```python
from build123d import *

# Parameters (mm, degrees)
SKETCH2_W     = 0.9
SKETCH2_H     = 0.2
CHAMFER1_SIZE = 0.8
CHAMFER2_SIZE = 0.3


with BuildPart() as part:
    # Sketch1 → Revolve1 (revolve)
    with BuildSketch(Plane(origin=(0, 0, 0), x_dir=(0, 0, -1), z_dir=(1, 0, 0)), mode=Mode.PRIVATE) as revolve1_sk:
        Polygon((-150, 0), (150, 0), (150, 4), (140, 4), (140, 6.32), (-96, 6.32), (-96, 4.94), (-135, 4.94), (-135, 4), (-150, 4), align=None)
    revolve(revolve1_sk.sketch.rotate(Axis((0, 0, 150), (0, 0, -1)), 90), axis=Axis((0, 0, 150), (0, 0, -1)))

    # Sketch2 → Cut-Revolve1 (revolve, cut)
    with BuildSketch(Plane(origin=(0, 0, 0), x_dir=(0, 0, -1), z_dir=(1, 0, 0)), mode=Mode.PRIVATE) as cut_revolve1_sk:
        with Locations((147.45, 3.9)):
            Rectangle(SKETCH2_W, SKETCH2_H)
    revolve(cut_revolve1_sk.sketch.rotate(Axis((0, 0, -150), (0, 0, 1)), 270), axis=Axis((0, 0, -150), (0, 0, 1)), mode=Mode.SUBTRACT)

    # Chamfer1
    chamfer1_edges = [part.edges().sort_by_distance(p)[0] for p in [
        (-4, 0, -150),
    ]]
    chamfer(chamfer1_edges, length=CHAMFER1_SIZE)

    # Chamfer2
    chamfer2_edges = [part.edges().sort_by_distance(p)[0] for p in [
        (-4.94, 0, 135),
        (-4, 0, 150),
    ]]
    chamfer(chamfer2_edges, length=CHAMFER2_SIZE)


solid = part.part
```
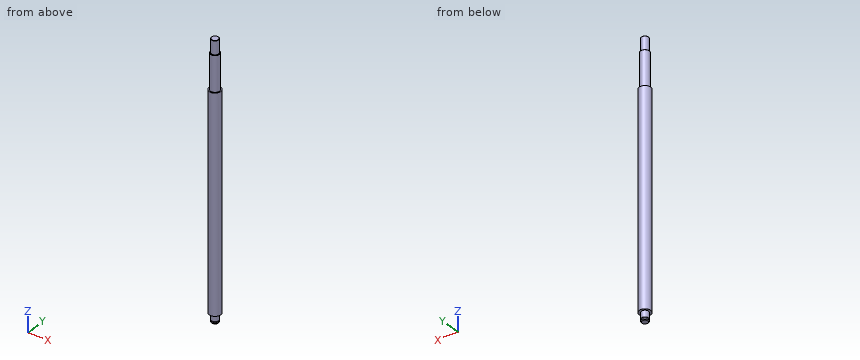
Geometry check sheet. Reference: the model listing, model coordinates, mm. Round coordinates to 2 decimals unless told otherwise and drop trailing zeros. Loops run counter-clockwise (first coordinate to the right, second up) from the corner with the lowest first, then second, coordinate; pieces in that order, holes last. Notation, with made-up numbers: M -23.5,-25.75 L 35.5,-25.75 A21 ccw 35.5,12.25 Z; hole C -15.75,21 d1. An arc over 180 degrees is marked long. Return JSON: item names as keys, results as strings. Group by question number.
(1) Go/stop test with flat-tipped pins: pin 1 (1.5 mm diameter, centred on y = -5, z = 114, fed in from -X); pin 2 (2 mm diameter, centred on y = 3.5, z = -95.5, fed in from -X); pin 3 (1 mm diameter, centred on x = 4.5, z = -66.5, fed in from +Y). Record where each tip stops, or that it passes through.
(2) Section check C-C, the plane z = 2. Enter the section's corners in (x, y), and give its area (3 significant figures).
(3) Scan lines: line 1 along Z through (x, y) = (-5, 0); line 2 along Z through (x, y) = (3.5, -3); line 3 along X through (y, z) = (0.5, 48). Record each from-to range of solid material in increasing order. Write a range as [from, to].
Data:
{
 "1": {"pin 1": "x = -2.52", "pin 2": "x = -5.8", "pin 3": "y = 4.89"},
 "2": {"outline": "C 0,0 d12.64", "area": "125 mm²"},
 "3": {"line 1": "[-140, 96]", "line 2": "[-140, 135]", "line 3": "[-6.3, 6.3]"}
}
